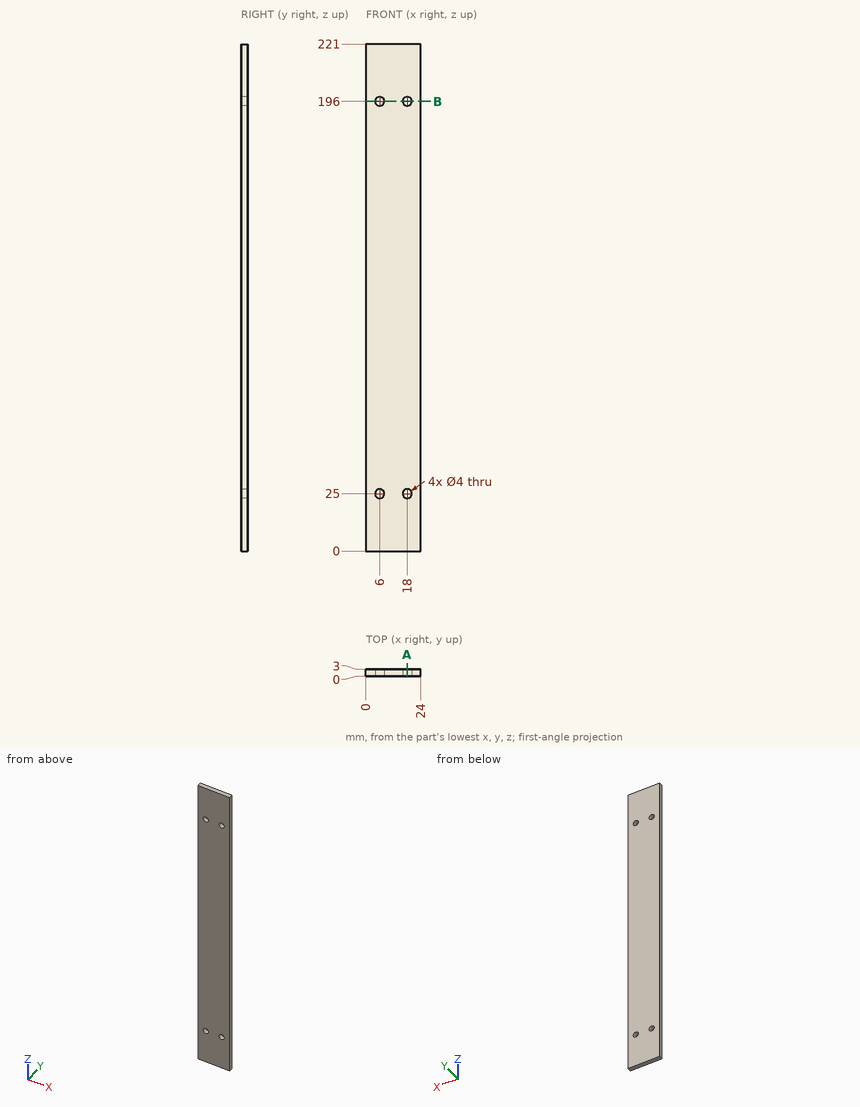
Input: dimensioned drawing with shaded views. Units: mm. Origin: part minimum x, y, z. Coordinates: 2 decimals unless noted, no trailing zeros. Order: outer loops, then holes, each group sorted by start corner. A loop starts at its lowest first (then second) coordinate and runs counter-clockwise, first axis right, second up.
Item 1: Material intervals for line 1 along Z through (x, y) = (6, 1.4); line 2 along X through (y, z) = (1.1, 196); line 3 along Z through (x, y) = (16.75, 2.65), sorted ascending.
Answer:
line 1: z = 0 to 23, 27 to 194, 198 to 221
line 2: x = 0 to 4, 8 to 16, 20 to 24
line 3: z = 0 to 23.44, 26.56 to 194.44, 197.56 to 221
Item 2: Section query A-A (x = 18). Output: boundary loops of the cut face in (y, z).
Answer:
outline: (0, 0) - (3, 0) - (3, 23) - (0, 23) - close; (0, 27) - (3, 27) - (3, 194) - (0, 194) - close; (0, 198) - (3, 198) - (3, 221) - (0, 221) - close
Item 3: Section query B-B (z = 196). Output: boundary loops of the cut face in (x, y).
Answer:
outline: (0, 0) - (4, 0) - (4, 3) - (0, 3) - close; (8, 0) - (16, 0) - (16, 3) - (8, 3) - close; (20, 0) - (24, 0) - (24, 3) - (20, 3) - close
